Part print with two shaded views. Sizes in mm from the minimum x, y, z corner. A direction names the side the tool comes from. Coordinates: 2 decimals unless noted, no trailing zeros. Loops run counter-clockwise (first coordinate to the right, second up) from the corner with the lowest first, then second, coordinate; pieces in that order, holes last. Notation, with made-up numbers: (6.25, -5.75) -> (30.25, -5.75) arc R17 cw to (30.25, 22.25) -> close; hole circle Ø1 at (-18.75, 10). An arc over 180 degrees is marked (long way). Answer as a JSON object with one key per item and string values. Group by question number.
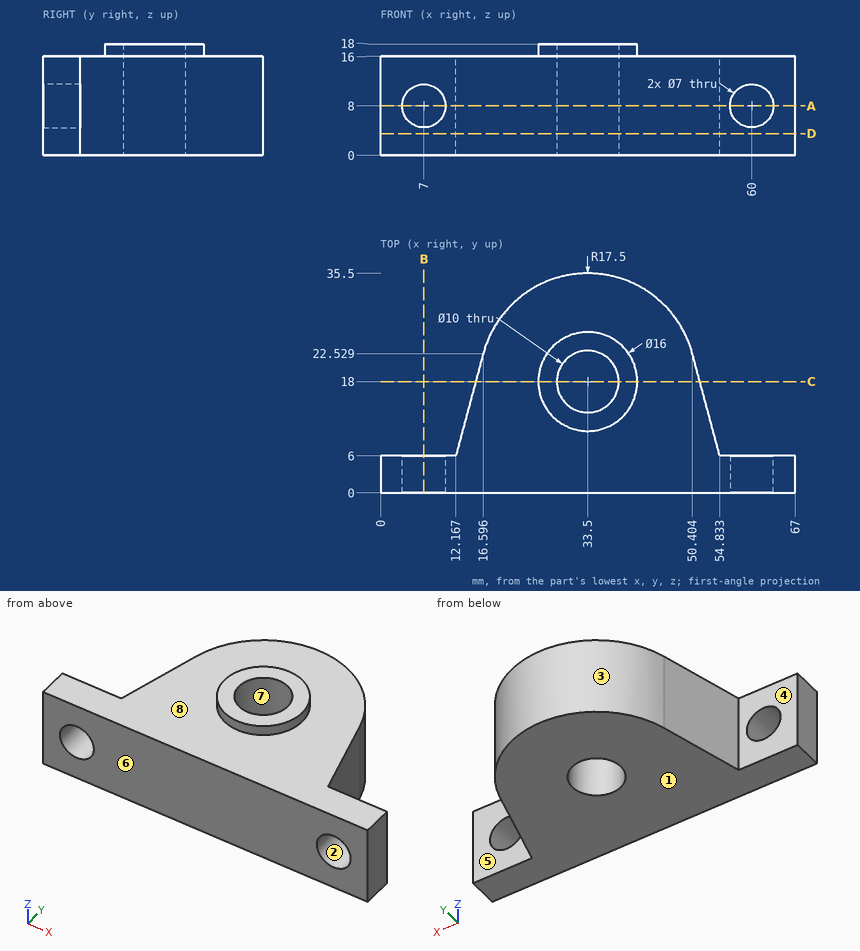
Item 1: Band-saw the part on B-B, the plane x = 7. List the corners of the cut face in (y, z), and give its area (3 significant figures).
Item 2: Pull direction X, two halves, no side cores. Call the marked faces 1, 2 and 3: +X half, -X half, draft (parallel to the pull), parting line (faces both ways), or undercut.
Item 3: Drill centre lines: L1, parallel to Z at x = 60, y = 3; L2, parallel to Z at x = 48.5, y = 24; L3, parallel to X at y = 20.5, z = 11. Where is each one in solid material? Low to high.
Item 4: Band-saw the part on D-D, the plane z = 3.5. List the corners of the cut face in (x, y).
Item 5: Flat gauge pins, fed straight in: P1, Ø2, axis at y = 10, z = 12, coming from the -X side; P2, Ø8, axis at y = 12, z = 6, coming from the +X side; P3, Ø3.5, axis at x = 9, z = 6.5, coming from the +Y side. Where does each tip first touch, or does it go through?
Item 6: Band-saw the part on C-C, the plane y = 18. List the corners of the cut face in (x, z).
Item 7: 3-axis set-ups, long thin cutter, end or side, ignore diameter. For the marked faces 4, 5, 6, 7 and 8: which of +Z, -Z, +X, -X, +Y, -Y reach the whole face in a straight line?
Item 8: Band-saw the part on A-A, the plane z = 8. List the corners of the cut face in (x, y).
Reply:
{
 "1": {"outline": "(0, 0) -> (6, 0) -> (6, 4.5) -> (0, 4.5) -> close; (0, 11.5) -> (6, 11.5) -> (6, 16) -> (0, 16) -> close", "area": "54.0 mm²"},
 "2": {"face 1": "draft", "face 2": "undercut", "face 3": "parting line"},
 "3": {"L1": "0 to 4.5, 11.5 to 16", "L2": "0 to 16", "L3": "16.05 to 29.17, 37.83 to 50.95"},
 "4": {"outline": "(0, 0) -> (67, 0) -> (67, 6) -> (54.83, 6) -> (50.4, 22.53) arc R17.5 ccw to (16.6, 22.53) -> (12.17, 6) -> (0, 6) -> close; hole circle Ø10 at (33.5, 18)"},
 "5": {"P1": "x = 12.97", "P2": "x = 54.3", "P3": "y = 6"},
 "6": {"outline": "(15.38, 0) -> (28.5, 0) -> (28.5, 18) -> (25.5, 18) -> (25.5, 16) -> (15.38, 16) -> close; (38.5, 0) -> (51.62, 0) -> (51.62, 16) -> (41.5, 16) -> (41.5, 18) -> (38.5, 18) -> close"},
 "7": {"face 4": "+Z, -Z, -X, +Y", "face 5": "+Z, -Z, +X, +Y", "face 6": "+Z, -Z, +X, -X, -Y", "face 7": "+Z, -Z", "face 8": "+Z"},
 "8": {"outline": "(0, 0) -> (3.5, 0) -> (3.5, 6) -> (0, 6) -> close; (10.5, 0) -> (56.5, 0) -> (56.5, 6) -> (54.83, 6) -> (50.4, 22.53) arc R17.5 ccw to (16.6, 22.53) -> (12.17, 6) -> (10.5, 6) -> close; (63.5, 0) -> (67, 0) -> (67, 6) -> (63.5, 6) -> close; hole circle Ø10 at (33.5, 18)"}
}
